Model file for the job. Use its own axes, mm. A direction names the side the tool comes from. Round coordinates to 2 decimals unless told otherwise and drop trailing zeros. Order: outer loops, then holes, each group sorted by start corner. A loop starts at its lowest first (then second) coordinate and runs counter-clockwise, first axis right, second up. Notation, with made-up numbers: (68, 44.25) - (94, 44.25) arc R17 ccw to (94, 75.25) - close; hole circle Ø4 at (-25.75, -18). An arc over 180 degrees is marked (long way). Use one line per item in the form item = value.
from build123d import *

# Parameters (mm, degrees)
SKETCH1_W           = 90
SKETCH1_H           = 20
SKETCH1_R           = 0.95
SKETCH1_W_2         = 18.3
SKETCH1_H_2         = 13
BOSS_EXTRUDE1_DEPTH = 5
CUT_EXTRUDE1_REACH  = 94.331
SKETCH3_R           = 1.25


with BuildPart() as part:
    # Sketch1 → Boss-Extrude1 (new body)
    with BuildSketch(Plane(origin=(0, 0, 0), x_dir=(1, 0, 0), z_dir=(0, 1, 0))):
        with Locations((45, 10)):
            Rectangle(SKETCH1_W, SKETCH1_H)
        with Locations(Location((57.88, 10, 0), (0, 0, 270))):
            Circle(SKETCH1_R, mode=Mode.SUBTRACT)
        with Locations(Location((60.98, 10, 0), (0, 0, 270))):
            Circle(SKETCH1_R, mode=Mode.SUBTRACT)
        with Locations(Location((64.08, 10, 0), (0, 0, 270))):
            Circle(SKETCH1_R, mode=Mode.SUBTRACT)
        with Locations(Location((67.18, 10, 0), (0, 0, 270))):
            Circle(SKETCH1_R, mode=Mode.SUBTRACT)
        with Locations(Location((70.28, 10, 0), (0, 0, 270))):
            Circle(SKETCH1_R, mode=Mode.SUBTRACT)
        with Locations(Location((19.72, 10, 0), (0, 0, 90))):
            Circle(SKETCH1_R, mode=Mode.SUBTRACT)
        with Locations(Location((22.82, 10, 0), (0, 0, 90))):
            Circle(SKETCH1_R, mode=Mode.SUBTRACT)
        with Locations(Location((25.92, 10, 0), (0, 0, 90))):
            Circle(SKETCH1_R, mode=Mode.SUBTRACT)
        with Locations(Location((29.02, 10, 0), (0, 0, 90))):
            Circle(SKETCH1_R, mode=Mode.SUBTRACT)
        with Locations(Location((32.12, 10, 0), (0, 0, 90))):
            Circle(SKETCH1_R, mode=Mode.SUBTRACT)
        with Locations((45, 10)):
            Rectangle(SKETCH1_W_2, SKETCH1_H_2, mode=Mode.SUBTRACT)
    extrude(amount=BOSS_EXTRUDE1_DEPTH)

    # Sketch3 → Cut-Extrude1 (cut, up to next)
    with BuildSketch(Plane(origin=(0, 5, 0), x_dir=(1, 0, 0), z_dir=(0, 1, 0)), mode=Mode.PRIVATE) as cut_extrude1_sk1:
        with Locations(Location((87, 3, 0), (0, 0, 270))):
            Circle(SKETCH3_R)
    cut_extrude1_tool1 = extrude(cut_extrude1_sk1.sketch, amount=-CUT_EXTRUDE1_REACH, mode=Mode.PRIVATE) & part.part
    # Sketch3 → Cut-Extrude1 (cut, up to next)
    with BuildSketch(Plane(origin=(0, 5, 0), x_dir=(1, 0, 0), z_dir=(0, 1, 0)), mode=Mode.PRIVATE) as cut_extrude1_sk2:
        with Locations(Location((79, 3, 0), (0, 0, 270))):
            Circle(SKETCH3_R)
    cut_extrude1_tool2 = extrude(cut_extrude1_sk2.sketch, amount=-CUT_EXTRUDE1_REACH, mode=Mode.PRIVATE) & part.part
    # Sketch3 → Cut-Extrude1 (cut, up to next)
    with BuildSketch(Plane(origin=(0, 5, 0), x_dir=(1, 0, 0), z_dir=(0, 1, 0)), mode=Mode.PRIVATE) as cut_extrude1_sk3:
        with Locations(Location((79, 17, 0), (0, 0, 90))):
            Circle(SKETCH3_R)
    cut_extrude1_tool3 = extrude(cut_extrude1_sk3.sketch, amount=-CUT_EXTRUDE1_REACH, mode=Mode.PRIVATE) & part.part
    # Sketch3 → Cut-Extrude1 (cut, up to next)
    with BuildSketch(Plane(origin=(0, 5, 0), x_dir=(1, 0, 0), z_dir=(0, 1, 0)), mode=Mode.PRIVATE) as cut_extrude1_sk4:
        with Locations(Location((87, 17, 0), (0, 0, 90))):
            Circle(SKETCH3_R)
    cut_extrude1_tool4 = extrude(cut_extrude1_sk4.sketch, amount=-CUT_EXTRUDE1_REACH, mode=Mode.PRIVATE) & part.part
    # Sketch3 → Cut-Extrude1 (cut, up to next)
    with BuildSketch(Plane(origin=(0, 5, 0), x_dir=(1, 0, 0), z_dir=(0, 1, 0)), mode=Mode.PRIVATE) as cut_extrude1_sk5:
        with Locations(Location((3, 17, 0), (0, 0, 270))):
            Circle(SKETCH3_R)
    cut_extrude1_tool5 = extrude(cut_extrude1_sk5.sketch, amount=-CUT_EXTRUDE1_REACH, mode=Mode.PRIVATE) & part.part
    # Sketch3 → Cut-Extrude1 (cut, up to next)
    with BuildSketch(Plane(origin=(0, 5, 0), x_dir=(1, 0, 0), z_dir=(0, 1, 0)), mode=Mode.PRIVATE) as cut_extrude1_sk6:
        with Locations(Location((11, 17, 0), (0, 0, 270))):
            Circle(SKETCH3_R)
    cut_extrude1_tool6 = extrude(cut_extrude1_sk6.sketch, amount=-CUT_EXTRUDE1_REACH, mode=Mode.PRIVATE) & part.part
    # Sketch3 → Cut-Extrude1 (cut, up to next)
    with BuildSketch(Plane(origin=(0, 5, 0), x_dir=(1, 0, 0), z_dir=(0, 1, 0)), mode=Mode.PRIVATE) as cut_extrude1_sk7:
        with Locations(Location((11, 3, 0), (0, 0, 90))):
            Circle(SKETCH3_R)
    cut_extrude1_tool7 = extrude(cut_extrude1_sk7.sketch, amount=-CUT_EXTRUDE1_REACH, mode=Mode.PRIVATE) & part.part
    # Sketch3 → Cut-Extrude1 (cut, up to next)
    with BuildSketch(Plane(origin=(0, 5, 0), x_dir=(1, 0, 0), z_dir=(0, 1, 0)), mode=Mode.PRIVATE) as cut_extrude1_sk8:
        with Locations(Location((3, 3, 0), (0, 0, 90))):
            Circle(SKETCH3_R)
    cut_extrude1_tool8 = extrude(cut_extrude1_sk8.sketch, amount=-CUT_EXTRUDE1_REACH, mode=Mode.PRIVATE) & part.part
    add(cut_extrude1_tool1.solids().sort_by_distance((87, 5, -3))[0], mode=Mode.SUBTRACT)
    add(cut_extrude1_tool2.solids().sort_by_distance((79, 5, -3))[0], mode=Mode.SUBTRACT)
    add(cut_extrude1_tool3.solids().sort_by_distance((79, 5, -17))[0], mode=Mode.SUBTRACT)
    add(cut_extrude1_tool4.solids().sort_by_distance((87, 5, -17))[0], mode=Mode.SUBTRACT)
    add(cut_extrude1_tool5.solids().sort_by_distance((3, 5, -17))[0], mode=Mode.SUBTRACT)
    add(cut_extrude1_tool6.solids().sort_by_distance((11, 5, -17))[0], mode=Mode.SUBTRACT)
    add(cut_extrude1_tool7.solids().sort_by_distance((11, 5, -3))[0], mode=Mode.SUBTRACT)
    add(cut_extrude1_tool8.solids().sort_by_distance((3, 5, -3))[0], mode=Mode.SUBTRACT)


solid = part.part
(1) Pull direction Z, two halves, no side cores. Call faces 3 (the face through (44, 2, 0)), 4 (the face through (90, 2, -10)), 5 (the face through (35.85, 2, -10)): released by +Z, released by -Z, zero draft, split by the parting line, or undercut.
Report:
face_3 = released by +Z
face_4 = zero draft
face_5 = undercut
(2) Slice it at D-D on z = -2.75. Give the cut face in (x, y), then the cut area to 3 significant figures.
Report:
outline = (0, 0) - (1.78, 0) - (1.78, 5) - (0, 5) - close; (4.22, 0) - (9.78, 0) - (9.78, 5) - (4.22, 5) - close; (12.22, 0) - (77.78, 0) - (77.78, 5) - (12.22, 5) - close; (80.22, 0) - (85.78, 0) - (85.78, 5) - (80.22, 5) - close; (88.22, 0) - (90, 0) - (90, 5) - (88.22, 5) - close
area = 401 mm2
(3) Probe probe 1 along Z at (x, y) = (87, 3.95); probe 2 along X at (y, z) = (3.6, -17); probe 3 along X at (y, z) = (1, -8.25). List the from-to ranges inside material, lowest first. Write a range as [from, to].
Report:
probe_1 = [-20, -18.25], [-15.75, -4.25], [-1.75, 0]
probe_2 = [0, 1.75], [4.25, 9.75], [12.25, 77.75], [80.25, 85.75], [88.25, 90]
probe_3 = [0, 35.85], [54.15, 90]
(4) Slice it at B-B on z = -12.5. Give the cut face in (x, y).
Report:
outline = (0, 0) - (35.85, 0) - (35.85, 5) - (0, 5) - close; (54.15, 0) - (90, 0) - (90, 5) - (54.15, 5) - close
(5) Tool access for faces 1 (the face through (44, 2, -20)), 2 (the face through (54.15, 2, -10)): list every direction of +Z, -Z, +X, -X, +Y, -Y with a clear straight run to the whole face (end or side of a thin tool).
Report:
face_1 = -Z, +X, -X, +Y, -Y
face_2 = +Y, -Y
(6) Slice it at C-C on y = 1.95. Count the separate pieces of the cut face and the enclosed holes in it, then the cut area to 3 significant figures.
Report:
separate_pieces = 1
enclosed_holes = 19
area = 1,490 mm2
(7) Pin check, flat tip, straight feed: pin 1 (1.5 mm diameter, centred on x = 57.88, z = -10, fed in from -Y). Stop position of the tip, or through.
Report:
pin_1 = through
(8) Slice it at A-A on x = 70.28. Give the cut face in (y, z).
Report:
outline = (0, -20) - (5, -20) - (5, -10.95) - (0, -10.95) - close; (0, -9.05) - (5, -9.05) - (5, 0) - (0, 0) - close
